```python
from build123d import *

# Parameters (mm, degrees)
F0_R     = 25
F0_R_2   = 20
F1_DEPTH = 20
F2_R     = 25
F3_DEPTH = 5
F4_R     = 2.5
F5_R     = 2.49999


# Not quite as in the source:
# - a fillet or chamfer is up to 0.001 mm smaller than in the source, because OpenCascade refuses the exact size


with BuildPart() as f1:
    # F0 (on Top) → F1 (new body)
    with BuildSketch(Plane.XY):
        Circle(F0_R)
        Circle(F0_R_2, mode=Mode.SUBTRACT)
    extrude(amount=F1_DEPTH)

    # F2 (on face) → F3 (join)
    with BuildSketch(Plane(origin=(0, 0, 0), x_dir=(1, 0, 0), z_dir=(0, 0, -1))):
        Circle(F2_R)
    extrude(amount=F3_DEPTH)

    # F4
    f4_edges = [f1.edges().sort_by_distance(p)[0] for p in [
        (-25, 0, 20),
    ]]
    fillet(f4_edges, radius=F4_R)

    # F5 (radius 2.5 in the source; OpenCascade refuses exactly that, so slightly less here)
    f5_edges = [f1.edges().sort_by_distance(p)[0] for p in [
        (-20, 0, 20),
    ]]
    fillet(f5_edges, radius=F5_R)


solid = f1.part
```
Here's how the part is built. I have some questions about the finished solid (model axes, mm). Give positions to 0.01 mm unless a question says otherwise; leave off trailing zeros. Order: outer loops, then holes, each group sorted by start corner. A loop starts at its lowest first (then second) coordinate and runs counter-clockwise, first axis right, second up. Notation, with made-up numbers: M -30,-6 L -2,-6 A23 ccw -2,14 Z; hole C 83,60.5 d5. An arc over 180 degrees is marked long. Use a Markdown table: item, result. Add a question column.
1. I need wall thicknesses on probe 1 along Y at (x, z) = (0, 7.75); probe 2 along Z at (x, y) = (-5.5, 10.5); probe 3 along Y at (x, z) = (-14, 1). Which ranges of each line are inside material? Lowest first, please. Write a range as from..to.
2. Suppose I cut it at C-C (z = 5.75). List the corners of the cut face in (x, y) for me.
3. For pin 1 Ø12 at (x, z) = (-8, 0.5) entering from +Y; pin 2 Ø6 at (y, z) = (-4.5, -1) entering from -X; pin 3 Ø12 at (x, y) = (5.5, 8.5) entering from +Z, each with a flat end and sliding along its axis, tell me the tip position at first contact or that it passes through.
4. If we mould it in two halves opening along X, with no side actions, what happens to faces 1 (the cylindrical face through (23.846, -7.509, 6.408)), 2 (the flat face through (0, 0, -5)), 3 (the cylindrical face through (-4.336, -19.524, 8.628))? For each: +X half, -X half, draft (parallel to the pull), parting line (faces both ways), or undercut.
Results list:
| question | item | result |
|---|---|---|
| 1 | probe 1 | y = -25..-20, 20..25 |
| 1 | probe 2 | z = -5..0 |
| 1 | probe 3 | y = -20.71..-14.28, 14.28..20.71 |
| 2 | outline | C 0,0 d50; hole C 0,0 d40 |
| 3 | pin 1 | stops at y = 24.92 |
| 3 | pin 2 | stops at x = -24.95 |
| 3 | pin 3 | stops at z = 0 |
| 4 | face 1 | parting line |
| 4 | face 2 | draft |
| 4 | face 3 | undercut |
